from build123d import *

# Parameters (mm, degrees)
SKETCH_W        = 50
SKETCH_H        = 56
PAD_DEPTH       = 12
SKETCH001_R     = 16.2
POCKET_DEPTH    = 12.001
PAD001_DEPTH    = 2
SKETCH004_W     = 72.31723
SKETCH004_H     = 2
POCKET001_DEPTH = 11.9
SKETCH005_W     = 25.040878
SKETCH005_H     = 17.68627
SKETCH005_W_2   = 12.208063
SKETCH005_H_2   = 50.590956
POCKET002_DEPTH = 5
SKETCH003_W     = 3
SKETCH003_H     = 6
POCKET003_DEPTH = 50.001
POCKET004_DEPTH = 35
FILLET_R        = 1.8
POCKET005_DEPTH = 20.001
CHAMFER_SIZE    = 3
FILLET001_R     = 5
FILLET002_R     = 5


with BuildPart() as part:
    # Sketch → Pad (new body)
    with BuildSketch(Plane.XY):
        Rectangle(SKETCH_W, SKETCH_H)
    extrude(amount=PAD_DEPTH)

    # Sketch001 → Pocket (cut, through all)
    with BuildSketch(Plane.XY.offset(12)):
        with Locations((0, -7.8)):
            Circle(SKETCH001_R)
    extrude(amount=-POCKET_DEPTH, mode=Mode.SUBTRACT)

    # Sketch009 → Pad001 (new body)
    with BuildSketch(Plane(origin=(0, 28, 0), x_dir=(-1, 0, 0), z_dir=(0, 1, 0))):
        Polygon((25, 12), (-34.464275, 20), (-34.464275, 0), (25, 0), align=None)
    extrude(amount=PAD001_DEPTH)

    # Sketch004 → Pocket001 (cut)
    with BuildSketch(Plane.XY.offset(12)):
        with Locations((-0.55157, -7.296643)):
            Rectangle(SKETCH004_W, SKETCH004_H)
    extrude(amount=-POCKET001_DEPTH, mode=Mode.SUBTRACT)

    # Sketch005 → Pocket002 (cut)
    with BuildSketch(Plane.XZ.offset(28)):
        with Locations((-27.520439, 4.662494)):
            Rectangle(SKETCH005_W, SKETCH005_H)
        with Locations((21.104031, -3.872155)):
            Rectangle(SKETCH005_W_2, SKETCH005_H_2)
    extrude(amount=-POCKET002_DEPTH, mode=Mode.SUBTRACT)

    # Sketch003 → Pocket003 (cut, through all)
    with BuildSketch(Plane.YZ.offset(25)):
        with Locations((-0.5, 6)):
            Rectangle(SKETCH003_W, SKETCH003_H)
    extrude(amount=-POCKET003_DEPTH, mode=Mode.SUBTRACT)

    # Sketch002 → Pocket004 (cut)
    with BuildSketch(Plane.XZ.offset(23)):
        Polygon((-22.5, 6), (-20.237258, 8.262742), (-17.974517, 6), (-20.237258, 3.737258), align=None)
        Polygon((17.974517, 6), (20.237258, 8.262742), (22.5, 6), (20.237258, 3.737258), align=None)
    extrude(amount=-POCKET004_DEPTH, mode=Mode.SUBTRACT)

    # Fillet
    fillet_edges = [part.edges().sort_by_distance(p)[0] for p in [
        (15, -28, 6),
        (15, -23, 6),
        (25, -23, 6),
        (-15, -28, 6),
        (-15, -23, 6),
        (-25, -23, 6),
    ]]
    fillet(fillet_edges, radius=FILLET_R)

    # Sketch010 → Pocket005 (cut, through all)
    with BuildSketch(Plane(origin=(0, 0, 0), x_dir=(1, 0, 0), z_dir=(0, 0, -1))):
        with BuildLine():
            ThreePointArc((-35.356641, -7.272038), (-13.77578, -26.704891), (13.751946, -35.956576))
            Line((13.751946, -35.956576), (-64.830559, -41.48777))
            Line((-64.830559, -41.48777), (-35.356641, -7.272038))
        make_face()
    extrude(amount=-POCKET005_DEPTH, mode=Mode.SUBTRACT)

    # Chamfer
    chamfer_edges = [part.edges().sort_by_distance(p)[0] for p in [
        (34.464275, 29, 0),
    ]]
    chamfer(chamfer_edges, length=CHAMFER_SIZE)

    # Fillet001
    fillet001_edges = [part.edges().sort_by_distance(p)[0] for p in [
        (34.464275, 29, 20),
    ]]
    fillet(fillet001_edges, radius=FILLET001_R)

    # Fillet002
    fillet002_edges = [part.edges().sort_by_distance(p)[0] for p in [
        (34.464275, 29, 3),
    ]]
    fillet(fillet002_edges, radius=FILLET002_R)


solid = part.part
Geometry check sheet. Reference: the model listing, model coordinates, mm. A direction names the side the tool comes from. Coordinates: 2 decimals unless noted, no trailing zeros. Order: outer loops, then holes, each group sorted by start corner. A loop starts at its lowest first (then second) coordinate and runs counter-clockwise, first axis right, second up. Notation, with made-up numbers: (74.25, -7) - (117.25, -7) arc R10 ccw to (117.25, 12) - close; hole circle Ø8 at (85, 2.5). An arc over 180 degrees is marked (long way). Answer in a Markdown table with one row per item. Add a question column.
1) Cross-section at B-B, the plane x = 0. Record the cut outline in (y, z).
2) Set-up check for faces 1 (the cylindrical face through (14.965, -14.005, 6.084)), 2 (the flat face through (34.464, 29, 10)), 3 (the flat face through (-18, 1, 5)), 4 (the flat face through (18.5, -23, 7.4)), 5 (the flat face through (19.122, 6.423, 4.853)): record each of +Z, -Z, +X, -X, +Y, -Y from which the full face is reachable in a straight line by a thin tool's end or side.
3) Cross-section at C-C, the plane z = 18.25. Record the cut outline in (x, y), then the cut area to 3 significant figures.
4) Release check for a two-part mould opening along Z. For faces 6 (the flat face through (20, 28, 14)), 7 (the flat face through (-19.09, -4.178, 4.884)), 8 (the cylindrical face through (34.1, 29, 3.2)) record: +Z half, -Z half, draft (parallel to the pull), parting line (faces both ways), or undercut.
5) Gauge pin test, flat ends, axial feed: P1, Ø3.5, axis at x = 21.5, z = 6, coming from the -Y side; P2, Ø7, axis at x = 19.5, z = 6, coming from the -Y side; P3, Ø6, axis at y = -5, z = 10.5, coming from the +X side. Record the tip position at first contact, or that the pin passes through.
6) Material ranges on line 1 along Y through (x, z) = (18, 8); line 2 along Y through (x, z) = (0, 8); line 3 along X through (y, z) = (-17.5, 4.75), recorded low to high. Write a range as [from, to].
7) Cross-section at A-A, the plane y = -10. Record the cut outline in (x, z), then the cut area to 3 significant figures.
8) Cross-section at D-D, the plane y = 26.5. Record the cut outline in (x, z), then the cut area to 3 significant figures.
Check result:
| question | item | result |
|---|---|---|
| 1 | outline | (-28, 0) - (-24, 0) - (-24, 12) - (-28, 12) - close; (8.4, 0) - (30, 0) - (30, 15.36) - (28, 15.36) - (28, 12) - (8.4, 12) - close |
| 2 | face 1 | +Z, -Z |
| 2 | face 2 | +Z, -Z, +X, +Y, -Y |
| 2 | face 3 | +X, -X |
| 2 | face 4 | +Z, -Z, +X, -Y |
| 2 | face 5 | -Y |
| 3 | outline | (21.46, 28) - (32.51, 28) - (32.51, 30) - (21.46, 30) - close |
| 3 | area | 22.1 mm² |
| 4 | face 6 | draft |
| 4 | face 7 | undercut |
| 4 | face 8 | -Z half |
| 5 | P1 | stops at y = -23 |
| 5 | P2 | stops at y = -23.19 |
| 5 | P3 | stops at x = 25 |
| 6 | line 1 | y = [-23, -8.3], [-6.3, -2], [1, 30] |
| 6 | line 2 | y = [-28, -24], [8.4, 30] |
| 6 | line 3 | x = [-25, -21.25], [-19.22, -12.97], [12.97, 19.22], [21.25, 25] |
| 7 | outline | (-25, 0) - (-16.05, 0) - (-16.05, 12) - (-25, 12) - close; (16.05, 0) - (25, 0) - (25, 12) - (16.05, 12) - close; hole (-22.5, 6) - (-20.24, 3.74) - (-17.97, 6) - (-20.24, 8.26) - close; hole (17.97, 6) - (20.24, 3.74) - (22.5, 6) - (20.24, 8.26) - close |
| 7 | area | 194 mm² |
| 8 | outline | (-14.12, 0) - (25, 0) - (25, 12) - (-14.12, 12) - close |
| 8 | area | 469 mm² |
